Check sheet for the modelled part. Datum: model origin and axes. Units: mm. A direction names the side the tool comes from. Give positions to 0.01 mm unless a question says otherwise; leave off trailing zeros. Order: outer loops, then holes, each group sorted by start corner. A loop starts at its lowest first (then second) coordinate and runs counter-clockwise, first axis right, second up.
Autodesk Inventor part; units mm, degrees
ref_plane "YZ Plane" through (0, 0, 0) normal (1, 0, 0) x (0, 1, 0)
ref_plane "XZ Plane" through (0, 0, 0) normal (0, 1, 0) x (-1, 0, 0)
ref_plane "XY Plane" through (0, 0, 0) normal (0, 0, 1) x (1, 0, 0)
sketch "Sketch1" plane through (0, 0, 0) normal (0, 1, 0) x (-1, 0, 0)
  line L0 (0, 0) -> (25.4, 0)
  line L1 (25.4, 0) -> (25.4, 101.6)
  line L2 (25.4, 101.6) -> (0, 101.6)
  line L3 (0, 101.6) -> (0, 0)
  circle A0 centre (12.7, 8.89) radius 3.5052
  circle A1 centre (6.1214, 8.89) radius 0.889
  circle A2 centre (19.2786, 8.89) radius 0.889
  line L4 (6.7, 62.71) -> (18.7, 62.71)
  line L5 (18.7, 62.71) -> (18.7, 92.71)
  line L6 (18.7, 92.71) -> (6.7, 92.71)
  line L7 (6.7, 92.71) -> (6.7, 62.71)
  circle A3 centre (12.7, 95.21) radius 1.0541
  circle A4 centre (12.7, 60.21) radius 1.0541
  dimension "d0" = 25.4
  dimension "d1" = 101.6
  dimension "d2" = 7.0104
  dimension "d3" = 8.89
  dimension "d4" = 12.7
  dimension "d5" = 1.778
  dimension "d6" = 1.778
  dimension "d7" = 13.1572
  dimension "d8" = 6.5786
  dimension "d9" = 8.89
  dimension "d10" = 8.89
  dimension "d11" = 12
  dimension "d12" = 30
  dimension "d13" = 8.89
  dimension "d14" = 6.7
  dimension "d15" = 2.1082
  dimension "d16" = 2.1082
  dimension "d17" = 6
  dimension "d18" = 6
  dimension "d19" = 35
  dimension "d20" = 2.5
extrude "Extrusion1" add sketch "Sketch1" along normal blind 3.175
equation "\"d0\" = armWidth"
equation "\"d1\" = armLength"
equation "\"d2\" = hornCenter"
equation "\"d3\" = hornOffset"
equation "\"d4\" = 0.5 * armWidth"
equation "\"d5\" = hornHole"
equation "\"d6\" = hornHole"
equation "\"d7\" = hornDia"
equation "\"d8\" = 0.5 * hornDia"
equation "\"d9\" = hornOffset"
equation "\"d10\" = hornOffset"
equation "\"d11\" = servoWidth"
equation "\"d12\" = servoLength"
equation "\"d13\" = servoOff"
equation "\"d14\" = -0.5 * servoWidth + 0.5 * armWidth"
equation "\"d15\" = servoHole"
equation "\"d16\" = servoHole"
equation "\"d17\" = 0.5 * servoWidth"
equation "\"d18\" = 0.5 * servoWidth"
equation "\"d19\" = servoDist"
equation "\"d20\" = -0.5 * servoLength + 0.5 * servoDist"
equation "\"d21\" = thick"
equation "\"thick\" = 3.175"
equation "\"hornCenter\" = 7.0104"
equation "\"hornDia\" = 13.1572"
equation "\"hornOffset\" = 8.89"
equation "\"hornHole\" = 1.778"
equation "\"servoLength\" = 30"
equation "\"servoWidth\" = 12"
equation "\"servoDist\" = 35"
equation "\"servoHole\" = 2.1082"
equation "\"servoOff\" = 8.89"
equation "\"armWidth\" = 25.4"
equation "\"armLength\" = 101.6"
properties part number "UpperArm"
Q1. Sectioned sample at C-C, the plane z = 8.89. Record the cut outline in (x, y) (3 decimals), plus the area to 3 significant figures.
Q2. Sectioned sample at A-A, the plane x = -17.5. Record the cut outline in (y, z) (3 decimals), plus the area to 3 significant figures.
Q3. Sectioned sample at B-B, the plane z = 95.21. Record the cut outline in (x, y) (3 decimals), plus the area to 3 significant figures.
Q4. Tool access check on faces 5 (the flat face through (-18.7, 2, 78)), 6 (the flat face through (-13, 2, 0)). Record the directions out of +Z, -Z, +X, -X, +Y, -Y that give a thin tool (end or side, any length) a straight path to the whole face; none if there is none.
Q5. Sectioned sample at D-D, the plane x = -12.7. Record the cut outline in (y, z) (3 decimals).
Q6. Material ranges on line 1 (Z direction, x = -12.7, y = 0.9); line 2 (X direction, y = 0.2, z = 90.5); line 3 (Z direction, x = -16.5, y = 2.55), recorded low to high.
Q7. Draft check along X on faces 1 (the cylindrical face through (-5.93, 1.57, 9.76)), 2 (the flat face through (0, 2, 52)), 3 (the cylindrical face through (-9.9, 1.6, 11)), 4 (the flat face through (-13, 2, 101.6)). Enter one of: pulls with the +X half, pulls with the -X half, needs draft (parallel to the pull), parting line crosses it, or undercut.
Filled in:
1. outline: (-25.4, 0) - (-20.168, 0) - (-20.168, 3.175) - (-25.4, 3.175) - close; (-18.39, 0) - (-16.205, 0) - (-16.205, 3.175) - (-18.39, 3.175) - close; (-9.195, 0) - (-7.01, 0) - (-7.01, 3.175) - (-9.195, 3.175) - close; (-5.232, 0) - (0, 0) - (0, 3.175) - (-5.232, 3.175) - close
1. area: 47.1 mm2
2. outline: (0, 0) - (3.175, 0) - (3.175, 62.71) - (0, 62.71) - close; (0, 92.71) - (3.175, 92.71) - (3.175, 101.6) - (0, 101.6) - close
2. area: 227 mm2
3. outline: (-25.4, 0) - (-13.754, 0) - (-13.754, 3.175) - (-25.4, 3.175) - close; (-11.646, 0) - (0, 0) - (0, 3.175) - (-11.646, 3.175) - close
3. area: 74.0 mm2
4. face 5: +Y, -Y
4. face 6: -Z, +X, -X, +Y, -Y
5. outline: (0, 0) - (3.175, 0) - (3.175, 5.385) - (0, 5.385) - close; (0, 12.395) - (3.175, 12.395) - (3.175, 59.156) - (0, 59.156) - close; (0, 61.264) - (3.175, 61.264) - (3.175, 62.71) - (0, 62.71) - close; (0, 92.71) - (3.175, 92.71) - (3.175, 94.156) - (0, 94.156) - close; (0, 96.264) - (3.175, 96.264) - (3.175, 101.6) - (0, 101.6) - close
6. line 1: z = 0 to 5.38, 12.4 to 59.16, 61.26 to 62.71, 92.71 to 94.16, 96.26 to 101.6
6. line 2: x = -25.4 to -18.7, -6.7 to 0
6. line 3: z = 0 to 62.71, 92.71 to 101.6
7. face 1: undercut
7. face 2: pulls with the +X half
7. face 3: undercut
7. face 4: needs draft
